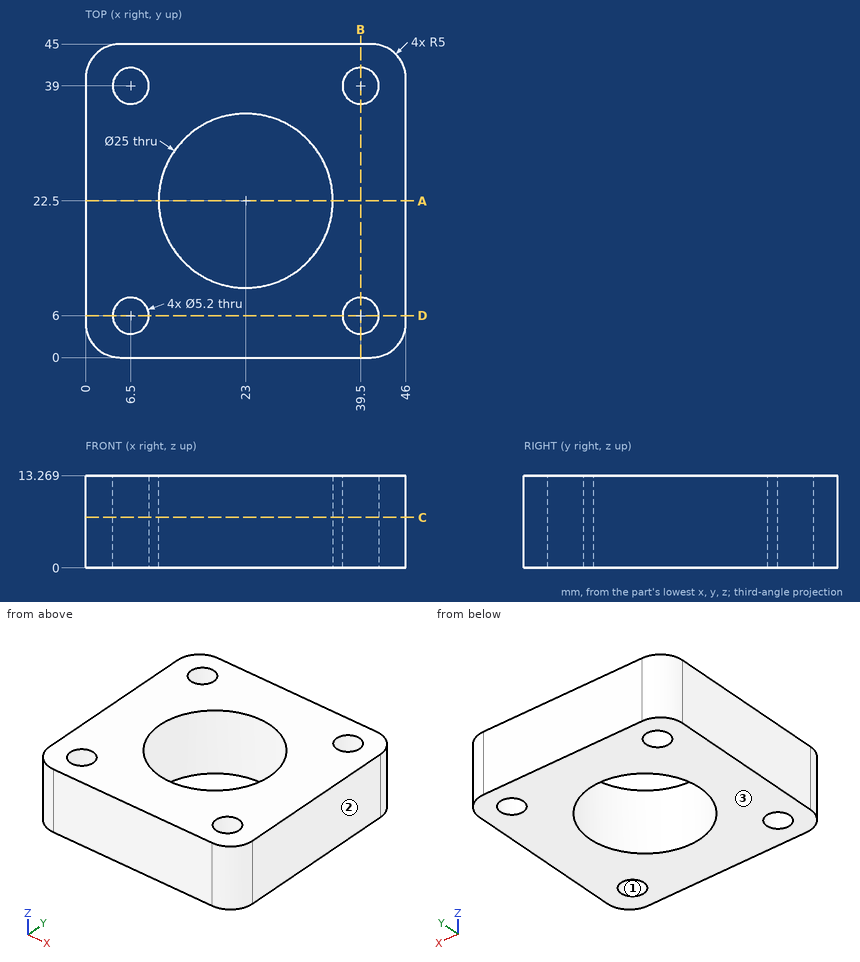
Print and shaded views of the part. All mm, measured from the part's lowest x, y and z. Coordinates: 2 decimals unless noted, no trailing zeros. Order: outer loops, then holes, each group sorted by start corner. A loop starts at its lowest first (then second) coordinate and runs counter-clockwise, first axis right, second up. Notation, with made-up numbers: (34, 36.25) - (52, 36.25) arc R19 cw to (52, 60.25) - close; hole circle Ø2 at (20.5, 21). An arc over 180 degrees is marked (long way). Return JSON: item names as keys, results as strings. Group by question number.
Item 1: Drill centre lines: probe 1 along X at (y, z) = (39, 6); probe 2 along Y at (x, z) = (39.5, 10); probe 3 along X at (y, z) = (4, 6.5). Where is each one in solid material? Low to high. Write a range as from..to.
Item 2: Cut at A-A (y = 22.5). List the corners of the cut face in (x, z), plus the area to 3 significant figures.
Item 3: Pull direction X, two halves, no side cores. Call the marked faces 1, 2 and 3: pulls with the +X half, pulls with the -X half, needs draft (parallel to the pull), parting line crosses it, or undercut.
Item 4: Cut at C-C (z = 7.25). List the corners of the cut face in (x, y), plus the area to 3 significant figures.
Item 5: Pin check, flat tips, straight feed: pin 1 (5 mm diameter, centred on y = 30, z = 9, fed in from -X); pin 2 (3 mm diameter, centred on x = 6.5, y = 39, fed in from -Z). Stop position of each tip, or through.
Item 6: Cut at B-B (x = 39.5). List the corners of the cut face in (y, z), plus the area to 3 significant figures.
Item 7: Cut at D-D (y = 6). List the corners of the cut face in (x, z).
Check values:
{
 "1": {"probe 1": "x = 0..3.9, 9.1..36.9, 42.1..46", "probe 2": "y = 0..3.4, 8.6..36.4, 41.6..45", "probe 3": "x = 0.1..4.84, 8.16..37.84, 41.16..45.9"},
 "2": {"outline": "(0, 0) - (10.5, 0) - (10.5, 13.27) - (0, 13.27) - close; (35.5, 0) - (46, 0) - (46, 13.27) - (35.5, 13.27) - close", "area": "279 mm2"},
 "3": {"face 1": "undercut", "face 2": "pulls with the +X half", "face 3": "needs draft"},
 "4": {"outline": "(0, 5) arc R5 ccw to (5, 0) - (41, 0) arc R5 ccw to (46, 5) - (46, 40) arc R5 ccw to (41, 45) - (5, 45) arc R5 ccw to (0, 40) - close; hole circle Ø5.2 at (6.5, 6); hole circle Ø5.2 at (6.5, 39); hole circle Ø25 at (23, 22.5); hole circle Ø5.2 at (39.5, 6); hole circle Ø5.2 at (39.5, 39)", "area": "1,470 mm2"},
 "5": {"pin 1": "stops at x = 0", "pin 2": "passes through"},
 "6": {"outline": "(0, 0) - (3.4, 0) - (3.4, 13.27) - (0, 13.27) - close; (8.6, 0) - (36.4, 0) - (36.4, 13.27) - (8.6, 13.27) - close; (41.6, 0) - (45, 0) - (45, 13.27) - (41.6, 13.27) - close", "area": "459 mm2"},
 "7": {"outline": "(0, 0) - (3.9, 0) - (3.9, 13.27) - (0, 13.27) - close; (9.1, 0) - (36.9, 0) - (36.9, 13.27) - (9.1, 13.27) - close; (42.1, 0) - (46, 0) - (46, 13.27) - (42.1, 13.27) - close"}
}
